Can you work these out from the model? Positions are in its coordinate system, mm. A direction names the side the tool comes from. Round coordinates to 2 decimals unless told otherwise and drop trailing zeros. Loops run counter-clockwise (first coordinate to the right, second up) from the corner with the lowest first, then second, coordinate; pieces in that order, holes last. Notation, with made-up numbers: M 14,-19.5 L 25,-19.5 A19 ccw 25,-14.5 Z; hole C 42,-3 d5. An arc over 180 degrees is marked long. Answer as CSV lines item,"result".
from build123d import *

# Parameters (mm, degrees)
SKETCH1_R               = 17.4625
SKETCH1_R_2             = 12.7
EXTRUDE_THIN1_DEPTH     = 152.4
CUT_EXTRUDE1_DEPTH      = 25.4
CUT_EXTRUDE1_DEPTH_BACK = 139.7
EXTRUDE_THIN2_DEPTH     = 6.35
SKETCH4_R               = 17.4625
BOSS_EXTRUDE1_DEPTH     = 2.54
FILLET1_R               = 2.54
BOSS_EXTRUDE2_START     = -0.185715
SKETCH5_W               = 5.08
SKETCH5_H               = 5.08
BOSS_EXTRUDE2_DEPTH     = 12.885715
CUT_EXTRUDE2_REACH      = 160.812
SKETCH6_W               = 7.62
SKETCH6_H               = 2.54
SKETCH7_R               = 1.27
CUT_EXTRUDE3_DEPTH      = 160.110904757


# Read off the part's stored shape, not the designer's step: Extrude-Thin2
with BuildPart() as part:
    # Sketch1 → Extrude-Thin1 (new body)
    with BuildSketch(Plane.XY):
        Circle(SKETCH1_R)
        Circle(SKETCH1_R_2, mode=Mode.SUBTRACT)
    extrude(amount=EXTRUDE_THIN1_DEPTH)

    # Sketch2 → Cut-Extrude1 (cut, two sides: drawn at the far end of the back side and taken through both)
    with BuildSketch(Plane(origin=(0, 0, 6.35), x_dir=(-1, 0, 0), z_dir=(0, 0, -1)).offset(-CUT_EXTRUDE1_DEPTH_BACK)):
        Polygon((-2.54, 2.54), (-31.75, 2.54), (-31.75, -2.54), (-2.54, -2.54), (-2.54, -31.75), (2.54, -31.75), (2.54, -2.54), (31.75, -2.54), (31.75, 2.54), (2.54, 2.54), (2.54, 31.75), (-2.54, 31.75), align=None)
    extrude(amount=CUT_EXTRUDE1_DEPTH + CUT_EXTRUDE1_DEPTH_BACK, mode=Mode.SUBTRACT)

    # Extrude-Thin2 outline → Extrude-Thin2 (add)
    with BuildSketch(Plane.XY):
        with BuildLine():
            Line((13.81111464, 2.51726107), (17.123388359, 2.51726107))
            ThreePointArc((17.123388359, 2.51726107), (20.0025, 0), (17.123388359, -2.51726107))
            Line((17.123388359, -2.51726107), (13.81111464, -2.51726107))
            Line((13.81111464, -2.51726107), (13.81111464, -2.54))
            Line((13.81111464, -2.54), (17.276785183, -2.54))
            ThreePointArc((17.276785183, -2.54), (17.17315149, -3.165718582), (17.046863636, -3.78726107))
            ThreePointArc((17.046863636, -3.78726107), (21.2725, 0), (17.046863636, 3.78726107))
            ThreePointArc((17.046863636, 3.78726107), (17.17315149, 3.165718582), (17.276785183, 2.54))
            Line((17.276785183, 2.54), (13.81111464, 2.54))
            Line((13.81111464, 2.54), (13.81111464, 2.51726107))
        make_face()
        with BuildLine():
            ThreePointArc((16.288020729, 6.295973871), (16.518015944, 5.665161561), (16.723590909, 5.025973871))
            ThreePointArc((16.723590909, 5.025973871), (22.5425, 0), (16.723590909, -5.025973871))
            ThreePointArc((16.723590909, -5.025973871), (16.518015944, -5.665161561), (16.288020729, -6.295973871))
            Line((16.288020729, -6.295973871), (16.635932996, -6.295973871))
            ThreePointArc((16.635932996, -6.295973871), (23.8125, 0), (16.635932996, 6.295973871))
            Line((16.635932996, 6.295973871), (16.288020729, 6.295973871))
        make_face()
        with BuildLine():
            ThreePointArc((-16.723590909, 5.025973871), (-16.518015944, 5.665161561), (-16.288020729, 6.295973871))
            Line((-16.288020729, 6.295973871), (-16.635932996, 6.295973871))
            ThreePointArc((-16.635932996, 6.295973871), (-23.8125, 0), (-16.635932996, -6.295973871))
            Line((-16.635932996, -6.295973871), (-16.288020729, -6.295973871))
            ThreePointArc((-16.288020729, -6.295973871), (-16.518015944, -5.665161561), (-16.723590909, -5.025973871))
            ThreePointArc((-16.723590909, -5.025973871), (-22.5425, 0), (-16.723590909, 5.025973871))
        make_face()
        with BuildLine():
            ThreePointArc((-17.276785183, 2.54), (-17.17315149, 3.165718582), (-17.046863636, 3.78726107))
            ThreePointArc((-17.046863636, 3.78726107), (-21.2725, 0), (-17.046863636, -3.78726107))
            ThreePointArc((-17.046863636, -3.78726107), (-17.17315149, -3.165718582), (-17.276785183, -2.54))
            Line((-17.276785183, -2.54), (-14.302412139, -2.54))
            Line((-14.302412139, -2.54), (-14.302412139, -2.51726107))
            Line((-14.302412139, -2.51726107), (-17.123388359, -2.51726107))
            ThreePointArc((-17.123388359, -2.51726107), (-20.0025, 0), (-17.123388359, 2.51726107))
            Line((-17.123388359, 2.51726107), (-14.302412139, 2.51726107))
            Line((-14.302412139, 2.51726107), (-14.302412139, 2.54))
            Line((-14.302412139, 2.54), (-17.276785183, 2.54))
        make_face()
    extrude(amount=EXTRUDE_THIN2_DEPTH)

    # Sketch4 → Boss-Extrude1 (add)
    with BuildSketch(Plane.XY.offset(152.4)):
        with Locations(Location((0, 0, 0), (0, 0, 171.636398211))):
            Circle(SKETCH4_R)
    extrude(amount=BOSS_EXTRUDE1_DEPTH)

    # Fillet1
    # the kernel refuses this fillet: 2.54 mm, written as the material it adds along each edge
    with BuildSketch(Plane(origin=(-16.288020729, -6.295973871, 0), x_dir=(0.3878333084832039, -0.9217295291087142, 0), z_dir=(0, 0, 1)), Plane(origin=(16.288020729, 6.295973871, 0), x_dir=(-0.38783330848320335, 0.9217295291087143, 0), z_dir=(0, 0, 1))) as fillet1_piece_1:
        with BuildLine():
            CenterArc((1.10244597, -2.53890008), FILLET1_R, 91.686230358, 27.467637925)
            Line((-0.134931966, -0.32068101), (-0.159679524, -0.276316629))
            ThreePointArc((-0.159679524, -0.276316629), (-0.114289843, -0.140638573), (-0.04682386, 0.019701932))
            Line((-0.04682386, 0.019701932), (0.001494842, 0.050778002))
            ThreePointArc((0.001494842, 0.050778002), (0.513851935, 0.043238053), (1.026209029, 0.050778002))
            Line((1.026209029, 0.050778002), (1.027703871, 0))
        make_face()
    extrude(amount=6.35)
    with BuildSketch(Plane(origin=(-16.288020729, 6.295973871, 0), x_dir=(0.38783330848320663, 0.9217295291087131, 0), z_dir=(0, 0, 1)), Plane(origin=(16.288020729, -6.295973871, 0), x_dir=(-0.3878333084832061, -0.9217295291087134, 0), z_dir=(0, 0, 1))) as fillet1_piece_2:
        with BuildLine():
            CenterArc((1.10244597, 2.53890008), FILLET1_R, 240.846131717, 27.467637925)
            Line((-0.134931966, 0.32068101), (-0.159679524, 0.276316629))
            ThreePointArc((-0.159679524, 0.276316629), (-0.114289843, 0.140638573), (-0.04682386, -0.019701932))
            Line((-0.04682386, -0.019701932), (0.001494842, -0.050778002))
            ThreePointArc((0.001494842, -0.050778002), (0.513851935, -0.043238053), (1.026209029, -0.050778002))
            Line((1.026209029, -0.050778002), (1.027703871, 0))
        make_face()
    extrude(amount=6.35)

    # Sketch5 → Boss-Extrude2 (add)
    with BuildSketch(Plane(origin=(17.4625, 0, 146.05), x_dir=(0, 0, -1), z_dir=(1, 0, 0)).offset(BOSS_EXTRUDE2_START)):
        with Locations((-6.35, 0)):
            Rectangle(SKETCH5_W, SKETCH5_H)
    boss_extrude2 = extrude(amount=BOSS_EXTRUDE2_DEPTH)

    # Sketch6 → Cut-Extrude2 (cut, up to next)
    with BuildSketch(Plane.XY.offset(154.94), mode=Mode.PRIVATE) as cut_extrude2_sk1:
        with Locations((26.3525, 0)):
            Rectangle(SKETCH6_W, SKETCH6_H)
    cut_extrude2_tool1 = extrude(cut_extrude2_sk1.sketch, amount=-CUT_EXTRUDE2_REACH, mode=Mode.PRIVATE) & part.part
    cut_extrude2 = cut_extrude2_tool1.solids().sort_by_distance((26.3525, 0, 154.94))[0]
    add(cut_extrude2, mode=Mode.SUBTRACT)

    # Sketch7 → Cut-Extrude3 (cut, through all)
    with BuildSketch(Plane.XZ.offset(2.54)):
        with Locations((27.6225, 152.4)):
            Circle(SKETCH7_R)
    cut_extrude3 = extrude(amount=-CUT_EXTRUDE3_DEPTH, mode=Mode.SUBTRACT)

    # Mirror2: Boss-Extrude2, Cut-Extrude2, Cut-Extrude3 across plane
    add(boss_extrude2.mirror(Plane(origin=(0, 0, 0), x_dir=(0, 0, 1), z_dir=(1, 0, 0))))
    add(cut_extrude2.mirror(Plane(origin=(0, 0, 0), x_dir=(0, 0, 1), z_dir=(1, 0, 0))), mode=Mode.SUBTRACT)
    add(cut_extrude3.mirror(Plane(origin=(0, 0, 0), x_dir=(0, 0, 1), z_dir=(1, 0, 0))), mode=Mode.SUBTRACT)


solid = part.part
Item 1: We'd pull the mould along Z, two halves only. Please class faces 5 (the face through (22, 0, 149.86)), 6 (the face through (-13, 3, 0)): released by +Z, released by -Z, zero draft, split by the parting line, or undercut.
Output:
face 5,"undercut"
face 6,"released by -Z"
Item 2: On a 3-axis mill with a long thin cutter (end or side, diameter ignored), from which of +Z, -Z, +X, -X, +Y, -Y can I reach the whole of each face in a straight line? I mean faces 1 (the face through (-24, 2.54, 152)), 2 (the face through (5.86, -11.267, 75.133)), 3 (the face through (24, -2.54, 152)), 4 (the face through (2.54, -15, 74)). Say none if no direction works.
Output:
face 1,"+Z, -X, +Y"
face 2,"-Z"
face 3,"+Z, +X, -Y"
face 4,"-Z, +Y, -Y"
Item 3: Will these pins go through, and if not, where does the flat tip stop? pin 1 (3 mm diameter, centred on y = -10, z = 75.5, fed in from -X); pin 2 (4 mm diameter, centred on x = 22, y = 1, fed in from -Z); pin 3 (1.4 mm diameter, centred on x = -15.5, z = 2.5, fed in from +Y); pin 4 (7.5 mm diameter, centred on x = 5.5, y = 1, fed in from -Z).
Output:
pin 1,"stops at x = -15.25"
pin 2,"stops at z = 0"
pin 3,"stops at y = 9.27"
pin 4,"stops at z = 152.4"
Item 4: If we section it at C-C on x = 9.5: Write out the boundary of the cut face in (y, z).
Output:
outline,"M -14.65,0 L -8.43,0 L -8.43,152.4 L 8.43,152.4 L 8.43,0 L 14.65,0 L 14.65,154.94 L -14.65,154.94 Z"
Item 5: If we section it at B-B on x = 0: Write out the boundary of the cut face in (y, z).
Output:
outline,"M -17.46,146.05 L -12.7,146.05 L -12.7,152.4 L 12.7,152.4 L 12.7,146.05 L 17.46,146.05 L 17.46,154.94 L -17.46,154.94 Z"
Item 6: If we section it at A-A on z = 52: Write out the boundary of the cut face in (x, y) (1 decimal), then the cut area to 3 significant figures.
Output:
outline,"M -17.3,-2.5 A17.5 ccw -2.5,-17.3 L -2.5,-12.4 A12.7 cw -12.4,-2.5 Z; M -17.3,2.5 L -12.4,2.5 A12.7 cw -2.5,12.4 L -2.5,17.3 A17.5 ccw Z; M 2.5,-17.3 A17.5 ccw 17.3,-2.5 L 12.4,-2.5 A12.7 cw 2.5,-12.4 Z; M 2.5,12.4 A12.7 cw 12.4,2.5 L 17.3,2.5 A17.5 ccw 2.5,17.3 Z"
area,"354 mm2"
Item 7: If I drill on line 1 along Z through (x, y) = (11, 6); line 2 along X through (y, z) = (14, 134); line 3 along X through (y, z) = (11, 64), over which ranges is the centre line in solid material (lowest first)? Write a range as from..to.
Output:
line 1,"z = 152.4..154.94"
line 2,"x = -10.44..-2.54, 2.54..10.44"
line 3,"x = -13.56..-6.35, 6.35..13.56"
